Read the model definition and answer for the solid it produces. Units are mm, in the model's axes. Round coordinates to 2 decimals unless told otherwise and drop trailing zeros. Write each loop counter-clockwise with the first axis right and the second up, starting at its lowest first coordinate (ties: lowest second). Pieces come first, ordered by that corner, then holes. Notation, with made-up numbers: (73, -8.5) -> (86, -8.5) arc R18 ccw to (86, 17.5) -> close; hole circle Ø5 at (15, 73.5). An arc over 180 degrees is marked (long way). Return JSON: item names as keys, results as strings.
from build123d import *

# Parameters (mm, degrees)
SKETCH1_W           = 18
SKETCH1_H           = 17
BOSS_EXTRUDE1_DEPTH = 2
SKETCH2_R           = 1.27
CUT_EXTRUDE1_DEPTH  = 3
FILLET1_R           = 2.54


with BuildPart() as part:
    # Sketch1 → Boss-Extrude1 (new body)
    with BuildSketch(Plane(origin=(0, 0, 0), x_dir=(1, 0, 0), z_dir=(0, 1, 0))):
        with Locations((9, 8.5)):
            Rectangle(SKETCH1_W, SKETCH1_H)
    extrude(amount=BOSS_EXTRUDE1_DEPTH)

    # Sketch2 → Cut-Extrude1 (cut, through all)
    with BuildSketch(Plane(origin=(0, 2, 0), x_dir=(1, 0, 0), z_dir=(0, 1, 0))):
        with Locations((2.54, 14.46)):
            Circle(SKETCH2_R)
        with Locations((15.46, 14.46)):
            Circle(SKETCH2_R)
    extrude(amount=-CUT_EXTRUDE1_DEPTH, mode=Mode.SUBTRACT)

    # Fillet1
    fillet1_edges = [part.edges().sort_by_distance(p)[0] for p in [
        (0, 1, -17),
        (18, 1, -17),
        (18, 1, 0),
        (0, 1, 0),
    ]]
    fillet(fillet1_edges, radius=FILLET1_R)


solid = part.part
Item 1: Section D-D (z = -0.75) is taken. Give the vertices of the cut face in (x, y).
Worked answers:
{"outline": "(0.74, 0) -> (17.26, 0) -> (17.26, 2) -> (0.74, 2) -> close"}
Item 2: Straight lines are drawn through the part: L1, parallel to X at y = 1.05, z = -14.46; L2, parallel to Z at x = 15.46, y = 0.5; L3, parallel to Z at x = 1.5, y = 1.6. For each, find the intervals that lie inside material, in ascending order. Write a range as [from, to].
Worked answers:
{"L1": "x = [0, 1.27], [3.81, 14.19], [16.73, 18]", "L2": "z = [-17, -15.73], [-13.19, 0]", "L3": "z = [-16.78, -15.19], [-13.73, -0.22]"}
Item 3: Section C-C (x = 16.25) is taken. Give the vertices of the cut face in (y, z).
Worked answers:
{"outline": "(0, -16.87) -> (2, -16.87) -> (2, -15.45) -> (0, -15.45) -> close; (0, -13.47) -> (2, -13.47) -> (2, -0.13) -> (0, -0.13) -> close"}
Item 4: Section A-A (y = 0.4) is taken. Give the vertices of the cut face in (x, z).
Worked answers:
{"outline": "(0, -14.46) arc R2.54 ccw to (2.54, -17) -> (15.46, -17) arc R2.54 ccw to (18, -14.46) -> (18, -2.54) arc R2.54 ccw to (15.46, 0) -> (2.54, 0) arc R2.54 ccw to (0, -2.54) -> close; hole circle Ø2.54 at (2.54, -14.46); hole circle Ø2.54 at (15.46, -14.46)"}
Item 5: Section B-B (x = 2.75) is taken. Give the vertices of the cut face in (y, z).
Worked answers:
{"outline": "(0, -17) -> (2, -17) -> (2, -15.71) -> (0, -15.71) -> close; (0, -13.21) -> (2, -13.21) -> (2, 0) -> (0, 0) -> close"}
